Check sheet for the drawn part. Datum: minimum x, y, z corner. Units: mm. Round coordinates to 2 decimals unless told otherwise and drop trailing zeros. Loops run counter-clockwise (first coordinate to the right, second up) from the corner with the lowest first, then second, coordinate; pieces in that order, holes last.
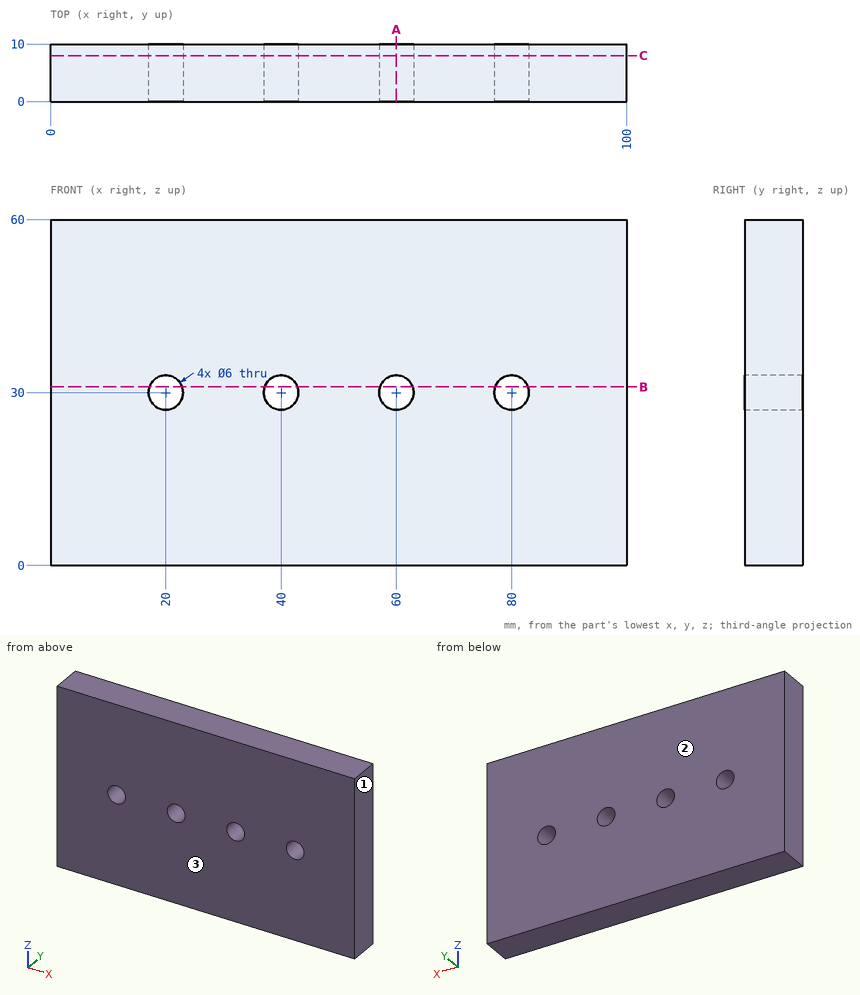
1) Sectioned sample at A-A, the plane x = 60. Record the cut outline in (y, z), then the cut area to 3 significant figures.
Report:
outline: (0, 0) - (10, 0) - (10, 27) - (0, 27) - close; (0, 33) - (10, 33) - (10, 60) - (0, 60) - close
area: 540 mm2
2) Gauge pin test, flat end, axial feed: pin 1 (5 mm diameter, centred on x = 60, z = 30, fed in from -Y). Record the tip position at first contact, or that the pin passes through.
Report:
pin 1: passes through
3) Mould release check, pull along Y, two halves, no side actions. Record for the marked faces 1, 2 and 3: +Y half, -Y half, draft (parallel to the pull), parting line (faces both ways), or undercut.
Report:
face 1: draft
face 2: +Y half
face 3: -Y half
4) Sectioned sample at C-C, the plane y = 8. Record the cut outline in (x, z).
Report:
outline: (0, 0) - (100, 0) - (100, 60) - (0, 60) - close; hole circle Ø6 at (20, 30); hole circle Ø6 at (40, 30); hole circle Ø6 at (60, 30); hole circle Ø6 at (80, 30)
5) Scan lines: line 1 along X through (y, z) = (5.25, 30); line 2 along Z through (x, y) = (40, 5.5); line 3 along Z through (x, y) = (41.5, 8.25). Record each from-to range of solid material in increasing order.
Report:
line 1: x = 0 to 17, 23 to 37, 43 to 57, 63 to 77, 83 to 100
line 2: z = 0 to 27, 33 to 60
line 3: z = 0 to 27.4, 32.6 to 60
6) Sectioned sample at B-B, the plane z = 31. Record the cut outline in (x, y), then the cut area to 3 significant figures.
Report:
outline: (0, 0) - (17.17, 0) - (17.17, 10) - (0, 10) - close; (22.83, 0) - (37.17, 0) - (37.17, 10) - (22.83, 10) - close; (42.83, 0) - (57.17, 0) - (57.17, 10) - (42.83, 10) - close; (62.83, 0) - (77.17, 0) - (77.17, 10) - (62.83, 10) - close; (82.83, 0) - (100, 0) - (100, 10) - (82.83, 10) - close
area: 774 mm2
